The drawing under review shows one solid part. Ordinate dimensions are in mm from its lowest x, y, z. A direction names the side the tool comes from. Round coordinates to 2 decimals unless told otherwise and drop trailing zeros. Order: outer loops, then holes, each group sorted by start corner. A loop starts at its lowest first (then second) coordinate and runs counter-clockwise, first axis right, second up.
1) Consider section C-C (z = 34). Give the boundary of the cut face in (x, y).
2) Clearance check with flat-ended pins moving along their axes: P1, Ø15, axis at x = 127.5, z = 424, coming from the +Y side; P2, Ø20.5, axis at y = 447, z = 176, coming from the +X side; P3, Ø12.5, axis at y = 442.5, z = 301.5, coming from the -X side. State where each tip first meets the part, or that it passes through.
3) To check wall thickness, follow L1, parallel to Z at x = 304, y = 424.5; L2, parallel to X at y = 347, z = 31. State the ranges of each line that lie inside material, in increasing order.
4) Consider section B-B (x = 177.5). Give the boundary of the cut face in (y, z), then the cut area to 3 significant figures.
5) Consider section D-D (y = 223.5). Give the boundary of the cut face in (x, z).
6) Machinability: for the marked faces 1, 2, 3 and 4, which of the approach directions +Z, -Z, +X, -X, +Y, -Y give a long, thin tool a straight path to every point of the face, cutting with its end or side? Answer none if there is none.
7) Consider section A-A (y = 32). Give the boundary of the cut face in (x, z), then the cut area to 3 significant figures.
8) Mouldability with a two-part tool opening along Z and no side actions: class the marked faces 5 and 6 as pulls with the +Z half, pulls with the -Z half, needs draft (parallel to the pull), parting line crosses it, or undercut.
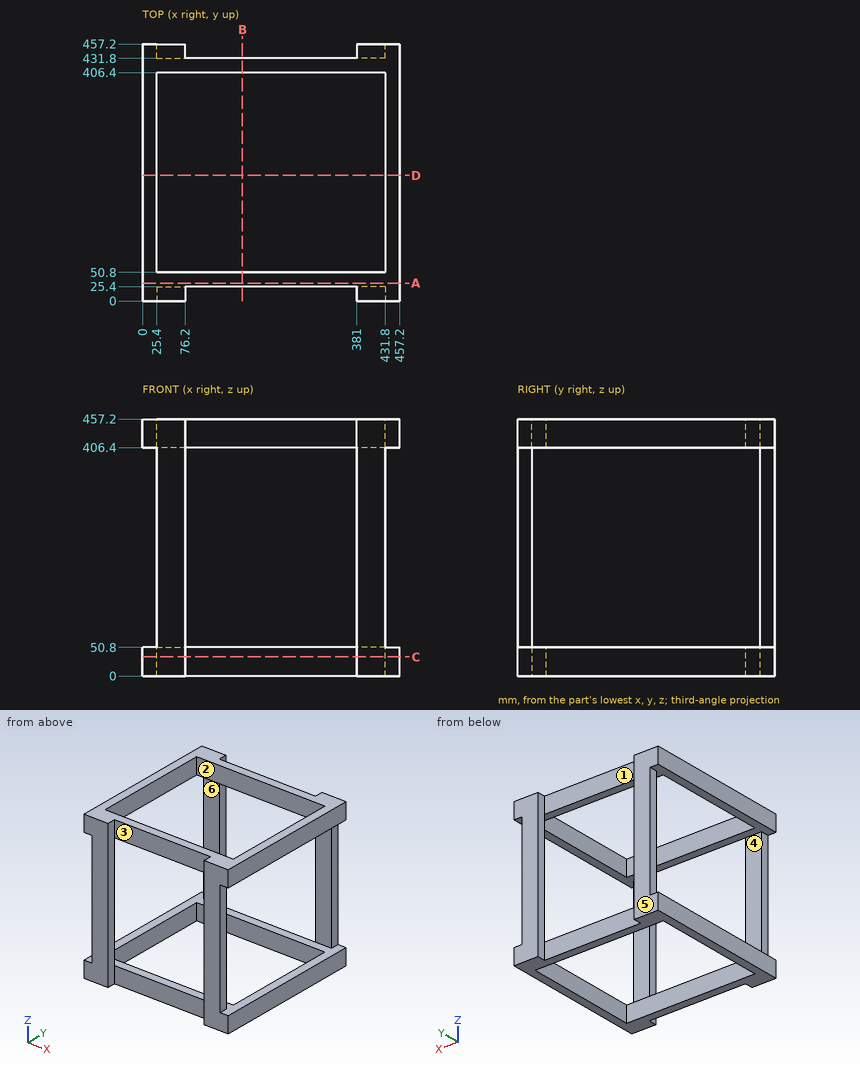
Answer below:
1. outline: (0, 0) - (76.2, 0) - (76.2, 25.4) - (381, 25.4) - (381, 0) - (457.2, 0) - (457.2, 457.2) - (381, 457.2) - (381, 431.8) - (76.2, 431.8) - (76.2, 457.2) - (0, 457.2) - close; hole (25.4, 50.8) - (431.8, 50.8) - (431.8, 406.4) - (25.4, 406.4) - close
2. P1: stops at y = 431.8
2. P2: stops at x = 431.8
2. P3: stops at x = 25.4
3. L1: z = 0 to 50.8, 406.4 to 457.2
3. L2: x = 0 to 25.4, 431.8 to 457.2
4. outline: (25.4, 0) - (50.8, 0) - (50.8, 50.8) - (25.4, 50.8) - close; (25.4, 406.4) - (50.8, 406.4) - (50.8, 457.2) - (25.4, 457.2) - close; (406.4, 0) - (431.8, 0) - (431.8, 50.8) - (406.4, 50.8) - close; (406.4, 406.4) - (431.8, 406.4) - (431.8, 457.2) - (406.4, 457.2) - close
4. area: 5,160 mm2
5. outline: (0, 0) - (25.4, 0) - (25.4, 50.8) - (0, 50.8) - close; (0, 406.4) - (25.4, 406.4) - (25.4, 457.2) - (0, 457.2) - close; (431.8, 0) - (457.2, 0) - (457.2, 50.8) - (431.8, 50.8) - close; (431.8, 406.4) - (457.2, 406.4) - (457.2, 457.2) - (431.8, 457.2) - close
6. face 1: +Z, -Z, +Y
6. face 2: +Z, -Z
6. face 3: +Z, -Z, -Y
6. face 4: +X, -X
7. outline: (0, 0) - (457.2, 0) - (457.2, 50.8) - (0, 50.8) - close; (0, 406.4) - (457.2, 406.4) - (457.2, 457.2) - (0, 457.2) - close
7. area: 46,500 mm2
8. face 5: needs draft
8. face 6: undercut
